```python
from build123d import *

# Parameters (mm, degrees)
BASE_FLANGE1_DEPTH = 2
EDGE_FLANGE1_DEPTH = 209.802637019
EDGE_FLANGE2_DEPTH = 208.43
CUT_EXTRUDE1_DEPTH = 10
CUT_EXTRUDE2_DEPTH = 10
CUT_EXTRUDE3_DEPTH = 10
CUT_EXTRUDE4_DEPTH = 10


# Sheet-metal steps are written as plain solids
with BuildPart() as part:
    # Sketch1 → Base-Flange1 (new body)
    with BuildSketch(Plane(origin=(0, 0, 0), x_dir=(1, 0, 0), z_dir=(0, 1, 0))):
        Polygon((0, 0), (208.43, 0), (208.43, 31.04), (0, 55), align=None)
    extrude(amount=-BASE_FLANGE1_DEPTH)

    # Edge-Flange1 section (across the edge) → Edge-Flange1 (add)
    with BuildSketch(Plane(origin=(0.084121612, -2, -55.731780783), x_dir=(-0.1142025683779395, -3.4914813388431334e-15, 0.9934574844329687), z_dir=(0.9934574844329687, 0, 0.1142025683779395))):
        with BuildLine():
            Line((-2, 0.7366), (-2, 8))
            Line((-2, 8), (0, 8))
            Line((0, 8), (0, 0.7366))
            ThreePointArc((0, 0.7366), (0.215745145, 0.215745145), (0.7366, 0))
            Line((0.7366, 0), (0.7366, -2))
            ThreePointArc((0.7366, -2), (-1.198468417, -1.198468417), (-2, 0.7366))
        make_face()
    extrude(amount=EDGE_FLANGE1_DEPTH)

    # Edge-Flange2 section (across the edge) → Edge-Flange2 (add)
    with BuildSketch(Plane(origin=(208.43, -2, 1.2766), x_dir=(0, 0, -1), z_dir=(-1, 0, 0))):
        with BuildLine():
            Line((-2, 0.7366), (-2, 8))
            Line((-2, 8), (0, 8))
            Line((0, 8), (0, 0.7366))
            ThreePointArc((0, 0.7366), (0.215745145, 0.215745145), (0.7366, 0))
            Line((0.7366, 0), (1.2766, 0))
            Line((1.2766, 0), (1.2766, -2))
            Line((1.2766, -2), (0.7366, -2))
            ThreePointArc((0.7366, -2), (-1.198468417, -1.198468417), (-2, 0.7366))
        make_face()
    extrude(amount=EDGE_FLANGE2_DEPTH)

    # Sketch12 → Cut-Extrude1 (cut)
    with BuildSketch(Plane(origin=(0, 0, 0), x_dir=(1, 0, 0), z_dir=(0, 1, 0))):
        Polygon((5, 54.425226695), (5, -0.54), (10, -0.54), (10, 53.85045339), align=None)
    extrude(amount=-CUT_EXTRUDE1_DEPTH, mode=Mode.SUBTRACT)

    # Sketch13 → Cut-Extrude2 (cut)
    with BuildSketch(Plane(origin=(0, 0, 0), x_dir=(1, 0, 0), z_dir=(0, 1, 0))):
        Polygon((15, 53.275680084), (15, -0.54), (20, -0.54), (20, 52.700906779), align=None)
        Polygon((25, 52.126133474), (25, -0.54), (30, -0.54), (30, 51.551360169), align=None)
        Polygon((35, 50.976586864), (35, -0.54), (40, -0.54), (40, 50.401813559), align=None)
        Polygon((45, 49.827040253), (45, -0.54), (50, -0.54), (50, 49.252266948), align=None)
    extrude(amount=-CUT_EXTRUDE2_DEPTH, mode=Mode.SUBTRACT)

    # Sketch14 → Cut-Extrude3 (cut)
    with BuildSketch(Plane(origin=(0, 0, 0), x_dir=(1, 0, 0), z_dir=(0, 1, 0))):
        Polygon((55, 48.677493643), (55, -0.54), (60, -0.54), (60, 48.102720338), align=None)
        Polygon((65, 47.527947033), (65, -0.54), (70, -0.54), (70, 46.953173727), align=None)
        Polygon((75, 46.378400422), (75, -0.54), (80, -0.54), (80, 45.803627117), align=None)
        Polygon((85, 45.228853812), (85, -0.54), (90, -0.54), (90, 44.654080507), align=None)
        Polygon((95, 44.079307201), (95, -0.54), (100, -0.54), (100, 43.504533896), align=None)
        Polygon((105, 42.929760591), (105, -0.54), (110, -0.54), (110, 42.354987286), align=None)
        Polygon((115, 41.780213981), (115, -0.54), (120, -0.54), (120, 41.205440676), align=None)
    extrude(amount=-CUT_EXTRUDE3_DEPTH, mode=Mode.SUBTRACT)

    # Sketch15 → Cut-Extrude4 (cut)
    with BuildSketch(Plane(origin=(0, 0, 0), x_dir=(1, 0, 0), z_dir=(0, 1, 0))):
        Polygon((125, 40.63066737), (125, -0.54), (130, -0.54), (130, 40.055894065), align=None)
        Polygon((135, 39.48112076), (135, -0.54), (140, -0.54), (140, 38.906347455), align=None)
        Polygon((145, 38.33157415), (145, -0.54), (150, -0.54), (150, 37.756800844), align=None)
        Polygon((155, 37.182027539), (155, -0.54), (160, -0.54), (160, 36.607254234), align=None)
        Polygon((165, 36.032480929), (165, -0.54), (170, -0.54), (170, 35.457707624), align=None)
        Polygon((175, 34.882934318), (175, -0.54), (180, -0.54), (180, 34.308161013), align=None)
        Polygon((185, 33.733387708), (185, -0.54), (190, -0.54), (190, 33.158614403), align=None)
        Polygon((195, 32.583841098), (195, -0.54), (200, -0.54), (200, 32.009067793), align=None)
    extrude(amount=-CUT_EXTRUDE4_DEPTH, mode=Mode.SUBTRACT)


solid = part.part
```
The listing builds one solid part. Answer for the finished solid, in the listing's coordinates (mm). A direction names the side the tool comes from. Give positions to 0.01 mm unless a question says otherwise; leave off trailing zeros. Write each loop counter-clockwise with the first axis right and the second up, starting at its lowest first coordinate (ties: lowest second). Pieces come first, ordered by that corner, then holes. Notation, with made-up numbers: (41.25, -38) -> (61.25, -38) arc R37 ccw to (61.25, 0) -> close; hole circle Ø6 at (34, -7). An arc over 180 degrees is marked (long way). Write item = value, one per line. Start each with the question number.
1) Straight lines are drawn through the part: line 1 along Z through (x, y) = (125.5, -0.5); line 2 along Z through (x, y) = (179, -7.75); line 3 along Y through (x, z) = (20.5, -8). For each, find the intervals that lie inside material, in ascending order.
2) The part is cut by section B-B, the plane z = -10. Count the separate pieces of the cut face and the enclosed holes in it, and give its area (3 significant figures).
3) The part is cut by section A-A, the plane y = -4.25. Determine the outline of the cut face in (x, z), and give its area (3 significant figures).
4) Each of these flat-tipped pins is pushed along its axis until it touches: pin 1 (2 mm diameter, centred on x = 45, y = -5.5, fed in from -Z); pin 2 (1.5 mm diameter, centred on x = 153.5, z = -19.5, fed in from -Y); pin 3 (1.6 mm diameter, centred on x = 108.5, y = -1, fed in from -Z); pin 4 (2 mm diameter, centred on x = 88.5, z = -31, fed in from -Y). Where does it stop, or does it pass through?
5) Which of the six approach directions +Z, -Z, +X, -X, +Y, -Y give full straight-line access (tool end or side, diameter ignored) to faces 1 (the face through (193, 0, -17)), 2 (the face through (143, -2, -19))?
6) Determine the mould class of faces 3 (the face through (43, -2, -25)), 4 (the face through (183, 0, -17)) for opening direction Z: +Z half, -Z half, draft (parallel to the pull), parting line (faces both ways), or undercut.
Solutions:
q1.line_1 = -42.16 to -40.57, 0.54 to 2.12
q1.line_2 = -37.18 to -35.16, 1.28 to 3.28
q1.line_3 = -2 to 0
q2.separate_pieces = 21
q2.enclosed_holes = 0
q2.area = 217 mm²
q3.outline = (0, 1.28) -> (208.43, 1.28) -> (208.43, 3.28) -> (0, 3.28) -> close; (0.08, -55.73) -> (0.31, -57.72) -> (208.74, -33.76) -> (208.51, -31.77) -> close
q3.area = 836 mm²
q4.pin_1 = -52.7
q4.pin_2 = -2
q4.pin_3 = -45.13
q4.pin_4 = through
q5.face_1 = +Z, -Z, +X, -X, +Y
q5.face_2 = -X, -Y
q6.face_3 = undercut
q6.face_4 = draft
